Build history of the part. All positions in model axes, mm. Face numbers are marked on the shaded views. Round coordinates to 2 decimals unless told otherwise and drop trailing zeros. Order: outer loops, then holes, each group sorted by start corner. A loop starts at its lowest first (then second) coordinate and runs counter-clockwise, first axis right, second up. Notation, with made-up numbers: (47, 35.5) -> (53, 35.5) arc R22 cw to (53, 71.5) -> close; hole circle Ø11 at (71, 65). An arc over 180 degrees is marked (long way). Write item = value, one per line.
from build123d import *

# Parameters (mm, degrees)
F0_R     = 4.364763
F1_DEPTH = 228.6
F2_R     = 4.118273
F2_R_2   = 7.189832
F2_R_3   = 4.635799
F3_DEPTH = 25.4


with BuildPart() as f1:
    # F0 (on Front) → F1 (new body)
    with BuildSketch(Plane.XZ):
        Polygon((-57.259552, 0), (0, 0), (0, 28.288946), (-1.533737, 28.288946), (-57.259552, 28.288946), align=None)
        with Locations((-30.504346, 11.929073)):
            Circle(F0_R, mode=Mode.SUBTRACT)
        Polygon((-40.047605, 44.478402), (-57.259552, 28.288946), (-1.533737, 28.288946), (-16.189458, 44.478402), align=None)
    extrude(amount=F1_DEPTH)

    # F2 (on face) → F3 (join)
    with BuildSketch(Plane.XY.offset(44.478402)):
        with Locations((-31.015592, -27.802045)):
            Circle(F2_R)
        with Locations((-31.015592, -55.409327)):
            Circle(F2_R_2)
        with Locations((-28.970607, -90.514891)):
            Circle(F2_R_3)
    extrude(amount=-F3_DEPTH)


solid = f1.part
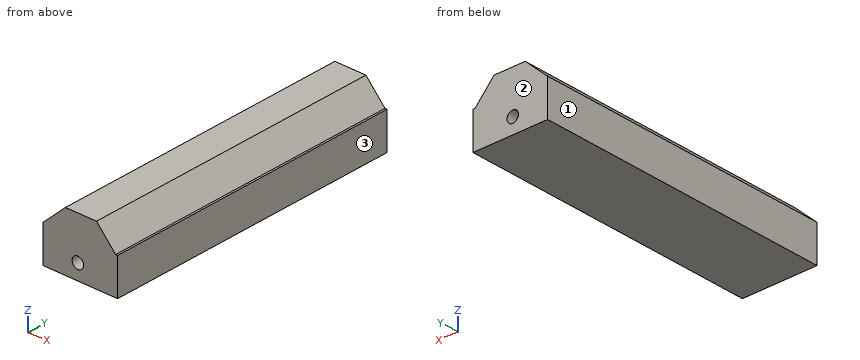
Q1. Cut at D-D, the plane z = 35. List the corners of the cut face in (x, y), and give its area (3 significant figures).
Check values:
outline = (-50.12, -228.6) -> (-7.61, -228.6) -> (-7.61, 0) -> (-50.12, 0) -> close
area = 9,720 mm²
Q2. Cut at B-B, the plane x = -32. List the corners of the cut face in (y, z), and give its area (3 significant figures).
Check values:
outline = (-228.6, 0) -> (0, 0) -> (0, 7.83) -> (-228.6, 7.83) -> close; (-228.6, 16.03) -> (0, 16.03) -> (0, 44.48) -> (-228.6, 44.48) -> close
area = 8,290 mm²
Q3. Mould opens along X. For the marked faces 1, 2 and 3 say: released by +X, released by -X, zero draft, split by the parting line, or undercut.
Check values:
face_1 = released by -X
face_2 = zero draft
face_3 = released by +X
Q4. Cut at C-C, the plane y = -188. List the corners of the cut face in (x, z), and give its area (3 significant figures).
Check values:
outline = (-57.26, 0) -> (0, 0) -> (0, 28.29) -> (-1.53, 28.29) -> (-16.19, 44.48) -> (-40.05, 44.48) -> (-57.26, 28.29) -> close; hole circle Ø8.73 at (-30.5, 11.93)
area = 2,200 mm²
Q5. Flat gauge pins, fed straight in: pin 1 (6 mm diameter, centred on y = -59.5, z = 33, fed in from +X); pin 2 (1.7 mm diameter, centred on x = -0.5, y = -164.5, fed in from +Z). Where does each tip first touch, or does it go through?
Check values:
pin_1 = -3.08
pin_2 = 28.29
Q6. Probe probe 1 along X at (y, z) = (-151, 11); probe 2 along X at (y, z) = (-141.5, 9); probe 3 along Z at (x, y) = (-16, -157.5). List the from-to ranges inside material, lowest first.
Check values:
probe_1 = -57.26 to -34.77, -26.24 to 0
probe_2 = -57.26 to -33.74, -27.27 to 0
probe_3 = 0 to 44.27
Q7. Cut at A-A, the plane z = 14. List the corners of the cut face in (x, y), and give its area (3 significant figures).
Check values:
outline = (-57.26, -228.6) -> (-34.35, -228.6) -> (-34.35, 0) -> (-57.26, 0) -> close; (-26.66, -228.6) -> (0, -228.6) -> (0, 0) -> (-26.66, 0) -> close
area = 11,300 mm²
